Autodesk Inventor part; units mm, degrees
ref_plane "YZ Plane" through (0, 0, 0) normal (1, 0, 0) x (0, 1, 0)
ref_plane "XZ Plane" through (0, 0, 0) normal (0, 1, 0) x (-1, 0, 0)
ref_plane "XY Plane" through (0, 0, 0) normal (0, 0, 1) x (1, 0, 0)
sketch "Sketch1" plane through (0, 0, 0) normal (0, 0, 1) x (1, 0, 0)
  line L0 (-76.2, -203.2) -> (76.2, -203.2)
  line L1 (76.2, -203.2) -> (76.2, 203.2)
  line L2 (76.2, 203.2) -> (-76.2, 203.2)
  line L3 (-76.2, 203.2) -> (-76.2, -203.2)
  line L4 (-76.2, -203.2) -> (76.2, 203.2) construction
  line L5 (76.2, -203.2) -> (-76.2, 203.2) construction
  point P0 (0, 0)
  dimension "d0" = 152.4
  dimension "d1" = 406.4
extrude "Plate1" add sketch "Sketch1" along normal blind 3.048
sketch "Sketch2" plane through (73.7032, 203.2, 1.7483) normal (0.819152, 0, -0.5735764) x (0, 1, 0)
  line L0 (-406.4, 0) -> (0, 0)
  line L1 (0, 0) -> (0, 508)
  line L2 (0, 508) -> (-406.4, 508)
  line L3 (-406.4, 508) -> (-406.4, 0)
edge flange "Flange1" height 508 angle 55 thickness 3.048 bend radius 3.048 thickness toward (0.819152, 0, -0.5735764) relief tear relief width 3.048 relief depth 1.524 corner gap 3.048 corner form 0 edges at (76.2, 0, 3.048) (-76.2, 0, 3.048) wall of the first edge with corners at (73.7032, -203.2, 1.7483) (73.7032, 203.2, 1.7483) (365.0801, 203.2, 417.8775) (365.0801, -203.2, 417.8775)
bend "Bend1"
corner "Corner1"
sketch "Sketch3" plane through (0, 0, 3.048) normal (0, 0, 1) x (1, 0, 0)
  line L0 (-78.0202, -203.2) -> (-78.0202, 152.4)
  line L1 (-78.0202, 152.4) -> (78.0202, 152.4)
  line L2 (78.0202, 152.4) -> (78.0202, -203.2)
  line L3 (-158.75, -203.2) -> (-78.0202, 152.4)
  line L4 (158.75, -203.2) -> (78.0202, 152.4)
  line L5 (-75.5234, -203.2) -> (-365.0801, -203.2)
  line L6 (75.5234, -203.2) -> (365.0801, -203.2)
  line L7 (-158.75, -203.2) -> (158.75, -203.2)
  line L8 (-78.0202, 203.2) -> (-78.0202, -203.2) construction
  line L9 (78.0202, -203.2) -> (78.0202, 203.2)
  line L10 (-73.0266, 203.2) -> (73.0266, 203.2)
  line L11 (73.0266, -203.2) -> (-73.0266, -203.2)
  point P0 (0, -203.2)
  point P1 (0, -203.2)
  dimension "d25" = 317.5
  dimension "d28" = 50.8
extrude "Cut1" cut sketch "Sketch3" against normal mid plane 508
sketch "Sketch4" plane through (0, 0, 3.048) normal (0, 0, 1) x (1, 0, 0)
  line L0 (-73.0266, 152.4) -> (73.0266, 152.4) construction
  line L1 (73.0266, 152.4) -> (73.0266, 203.2) construction
  line L2 (-73.0266, 203.2) -> (73.0266, 203.2) construction
  line L3 (-73.0266, 203.2) -> (-73.0266, 152.4) construction
  line L4 (0, 203.2) -> (0, 152.4) construction
  line L5 (0, 190.5) -> (6.35, 190.5)
  point P0 (0, 0)
  point P1 (-6.35, 190.5)
  dimension "d16" = 6.35
  dimension "d17" = 12.7
hole "Hole1" at (6.35, 190.5, 3.048) at (-6.35, 190.5, 3.048) direction (0, 0, -1) diameter 5.1054 end through all
equation "\"d23\" = Thickness"
equation "\"d2\" = Thickness"
equation "\"d3\" = BendReliefWidth"
equation "\"d4\" = BendReliefDepth"
equation "\"d5\" = MinimumRemnant"
equation "\"d6\" = TransitionRadius"
equation "\"d9\" = BendRadius"
equation "\"d10\" = CornerReliefSize"
equation "\"d11\" = GapSize"
equation "\"d12\" = JacobiRadiusSize"
equation "\"BendRadius\" = Thickness"
equation "\"BendReliefWidth\" = Thickness"
equation "\"BendReliefDepth\" = 0.5 * Thickness"
equation "\"CornerReliefSize\" = 4 * Thickness"
equation "\"MinimumRemnant\" = 2 * Thickness"
equation "\"TransitionRadius\" = BendRadius"
equation "\"JacobiRadiusSize\" = BendRadius"
equation "\"GapSize\" = Thickness"
properties part number "hopper" material "Polycarbonate, Smoke"
Input: part model. Units: mm. Frame: model coordinates. A direction names the side the tool comes from. Give positions to 0.01 mm unless a question says otherwise; leave off trailing zeros. Order: outer loops, then holes, each group sorted by start corner. A loop starts at its lowest first (then second) coordinate and runs counter-clockwise, first axis right, second up.
Q1. Contact query for flat-ended pins moving along their axis: pin 1 Ø1.5 at (y, z) = (124, 313.5) entering from -X; pin 2 Ø1.5 at (y, z) = (28.5, 170.5) entering from +X; pin 3 Ø12 at (y, z) = (117.5, 154) entering from -X. Output: stop coordinate, or through.
Checked values:
pin 1: stops at x = -296.24
pin 2: stops at x = 196.11
pin 3: stops at x = -188.23
Q2. Draft query along X for faces 1 (the flat face through (-263, -203.2, 269)), 2 (the flat face through (-224.825, -2.845, 212.259)), 3 (the flat face through (-118.573, -26.23, 63.185)), 4 (the flat face through (224.825, 2.845, 212.259)). Return one class per face: +X half, -X half, draft (parallel to the pull), parting line (faces both ways), or undercut.
Checked values:
face 1: draft
face 2: -X half
face 3: undercut
face 4: +X half
Q3. Section C-C on x = -234.5. Output: boundary loops of the cut face in (y, z), and give its area (3 significant figures).
Checked values:
outline: (-203.2, 226.08) - (203.2, 226.08) - (203.2, 231.39) - (-203.2, 231.39) - close
area: 2,160 mm2
Q4. Section B-B on z = 247.5. Output: boundary loops of the cut face in (x, y).
Checked values:
outline: (-249.5, -203.2) - (-245.78, -203.2) - (-245.78, 203.2) - (-249.5, 203.2) - close; (245.78, -203.2) - (249.5, -203.2) - (249.5, 203.2) - (245.78, 203.2) - close
Q5. Section D-D on x = -109.5. Output: boundary loops of the cut face in (y, z), and give its area (3 significant figures).
Checked values:
outline: (13.74, 47.56) - (203.2, 47.56) - (203.2, 52.87) - (13.74, 52.87) - close
area: 1,010 mm2
Q6. Section A-A on y = -115. Output: boundary loops of the cut face in (x, z).
Checked values:
outline: (-367.58, 416.13) - (-138.73, 89.3) - (-138.73, 94.61) - (-365.08, 417.88) - close; (138.73, 89.3) - (367.58, 416.13) - (365.08, 417.88) - (138.73, 94.61) - close
Q7. Ray query, probe 1 along Y at (x, z) = (-6.35, 2.3); probe 2 along X at (y, z) = (190.5, 1.85); probe 3 along X at (y, z) = (190.5, 0.95). Return the intervals inside material, ascending.
Checked values:
probe 1: y = 152.4 to 187.95, 193.05 to 203.2
probe 2: x = -77.4 to -8.9, -3.8 to 3.8, 8.9 to 77.4
probe 3: x = -76.29 to -8.9, -3.8 to 3.8, 8.9 to 76.29
Q8. Set-up query: faces 5 (the flat face through (118.573, -26.23, 63.185)), 6 (the flat face through (-1, 178, 3.048)), 7 (the flat face through (-1, 178, 0)). Return all of +Z, -Z, +X, -X, +Y, -Y with unobstructed straight access to the full face (end or side cutting, diameter ignored); none if empty.
Checked values:
face 5: +Z, -Z, -Y
face 6: +Z, +Y, -Y
face 7: -Z, +X, -X, +Y, -Y
